Geometry check sheet. Reference: the model listing, model coordinates, mm. A direction names the side the tool comes from. Give positions to 0.01 mm unless a question says otherwise; leave off trailing zeros. Loops run counter-clockwise (first coordinate to the right, second up) from the corner with the lowest first, then second, coordinate; pieces in that order, holes last. Notation, with made-up numbers: (2.25, -24) -> (6.25, -24) arc R18 cw to (6.25, -4) -> close; hole circle Ø5 at (46.5, -26). An arc over 180 degrees is marked (long way). Write each question's results on one line, items separated by ' | '. Start each with the question number.
1) Depth check by flat-ended pin: pin 1 (1.5 mm diameter, centred on y = 0, z = 1.5, fed in from -X); pin 2 (2 mm diameter, centred on y = 1.5, z = 2.5, fed in from -X); pin 3 (1.5 mm diameter, centred on x = 3.5, y = -0.5, fed in from -Z). Enter the tip coordinate at first touch or a pass-through.
2) Sectioned sample at A-A on z = 0. Record the cut outline in (x, y).
3) Draft check along Z on faces 1 (the face through (-3, 0, 0)), 2 (the face through (0, 0, -1)), 3 (the face through (-0.1, 1.5, 7.25)), 4 (the face through (1, -2, -1)). Enter one of: pulls with the +Z half, pulls with the -Z half, needs draft (parallel to the pull), parting line crosses it, or undercut.
4) Sectioned sample at B-B on x = 0. Record the cut outline in (y, z).
5) Set-up check for faces 5 (the face through (0.1, 1, 3.3)), 6 (the face through (9.736, 1.493, -0.114)): record each of +Z, -Z, +X, -X, +Y, -Y from which the full face is reachable in a straight line by a thin tool's end or side.
6) Scan lines: line 1 (Z direction, x = 0, y = -0.7); line 2 (Y direction, x = 2.5, z = -2); line 3 (Z direction, x = 2.5, y = -1.65). Record each from-to range of solid material in increasing order. Write a range as from..to.
7) Sectioned sample at D-D on z = -4.75. Record the cut outline in (x, y), then the cut area to 3 significant figures.
8) Sectioned sample at C-C on y = 0.7. Record the cut outline in (x, z), then the cut area to 3 significant figures.
```python
from build123d import *

# Parameters (mm, degrees)
SKETCH255_AS_DRAWN_R                 = 1
EXTRUDE056_DEPTH                     = 5
EXTRUDE056_ONTO_SKETCH255_ROLL_ANGLE = 90
SKETCH254_AS_DRAWN_R                 = 3
EXTRUDE057_DEPTH                     = 3
EXTRUDE057_ONTO_SKETCH254_ROLL_ANGLE = 90
FILLET003_R                          = 0.5
EXTRUDE048_DEPTH                     = 1
EXTRUDE048_ONTO_SKETCH245_ROLL_ANGLE = 90


with BuildPart() as extrude056:
    # Sketch255 as drawn → Extrude056 (new)
    with BuildSketch(Plane.XY):
        Circle(SKETCH255_AS_DRAWN_R)
    extrude(amount=-EXTRUDE056_DEPTH)


with BuildPart() as extrude056_1:
    # Extrude056 onto Sketch255 roll: moved
    add(extrude056.part.rotate(Axis((0, 0, 0), (1, 0, 0)), EXTRUDE056_ONTO_SKETCH255_ROLL_ANGLE))


with BuildPart() as extrude056_2:
    # Extrude056 onto Sketch255 placement: moved
    add(extrude056_1.part.moved(Location((0, -3, 0))))


with BuildPart() as fillet003:
    # Sketch254 as drawn → Extrude057 (new)
    with BuildSketch(Plane.XY):
        Circle(SKETCH254_AS_DRAWN_R)
    extrude(amount=-EXTRUDE057_DEPTH)


with BuildPart() as fillet003_1:
    # Extrude057 onto Sketch254 roll: moved
    add(fillet003.part.rotate(Axis((0, 0, 0), (1, 0, 0)), EXTRUDE057_ONTO_SKETCH254_ROLL_ANGLE))


with BuildPart() as fillet003_2:
    # Extrude057 onto Sketch254 placement: moved
    add(fillet003_1.part.moved(Location((0, -2.5, 0))))


with BuildPart() as fillet003_3:
    # Extrude057 placement: moved
    add(fillet003_2.part.moved(Location((0, 0.5, 0))))

    # Fillet003
    fillet003_edges = [fillet003_3.edges().sort_by_distance(p)[0] for p in [
        (-3, -2, 0),
    ]]
    fillet(fillet003_edges, radius=FILLET003_R)


with BuildPart() as cut034:
    # Sketch245 as drawn → Extrude048 (new)
    with BuildSketch(Plane.XY):
        with BuildLine():
            Line((-6.5, 7.250002), (6.499997, 7.250002))
            ThreePointArc((6.499997, -7.250002), (9.737171, 0), (6.499997, 7.250002))
            Line((-6.5, -7.250002), (6.499997, -7.250002))
            ThreePointArc((-6.5, 7.250002), (-9.737172, 0), (-6.5, -7.250002))
        make_face()
    extrude(amount=-EXTRUDE048_DEPTH)


with BuildPart() as cut034_1:
    # Extrude048 onto Sketch245 roll: moved
    add(cut034.part.rotate(Axis((0, 0, 0), (1, 0, 0)), EXTRUDE048_ONTO_SKETCH245_ROLL_ANGLE))


with BuildPart() as cut034_2:
    # Extrude048 onto Sketch245 placement: moved
    add(cut034_1.part)


with BuildPart() as cut034_3:
    # Extrude048 placement: moved
    add(cut034_2.part.moved(Location((0, 1, 0))))

    # Fusion018: union Fillet003
    add(fillet003_3.part)

    # Cut034: cut Extrude056
    add(extrude056_2.part, mode=Mode.SUBTRACT)


solid = cut034_3.part
```
Result:
1) pin 1: x = -2.9 | pin 2: x = -9.62 | pin 3: z = -1.2
2) outline: (-9.74, 1) -> (-3, 1) -> (-3, -1.5) arc R0.5 ccw to (-2.5, -2) -> (-1, -2) -> (-1, 2) -> (-9.74, 2) -> close; (1, -2) -> (2.5, -2) arc R0.5 ccw to (3, -1.5) -> (3, 1) -> (9.74, 1) -> (9.74, 2) -> (1, 2) -> close
3) face 1: parting line crosses it | face 2: undercut | face 3: pulls with the +Z half | face 4: needs draft
4) outline: (-2, -2.5) arc R0.5 ccw to (-1.5, -3) -> (1, -3) -> (1, -7.25) -> (2, -7.25) -> (2, -1) -> (-2, -1) -> close; (-2, 1) -> (2, 1) -> (2, 7.25) -> (1, 7.25) -> (1, 3) -> (-1.5, 3) arc R0.5 ccw to (-2, 2.5) -> close
5) face 5: -Y | face 6: +X, +Y, -Y
6) line 1: -3..-1, 1..3 | line 2: 1..2 | line 3: -1.62..1.62
7) outline: (-8.5, 1) -> (8.5, 1) -> (8.5, 2) -> (-8.5, 2) -> close | area: 17.0 mm^2
8) outline: circle Ø6 at (0, 0); hole circle Ø2 at (0, 0) | area: 25.1 mm^2
